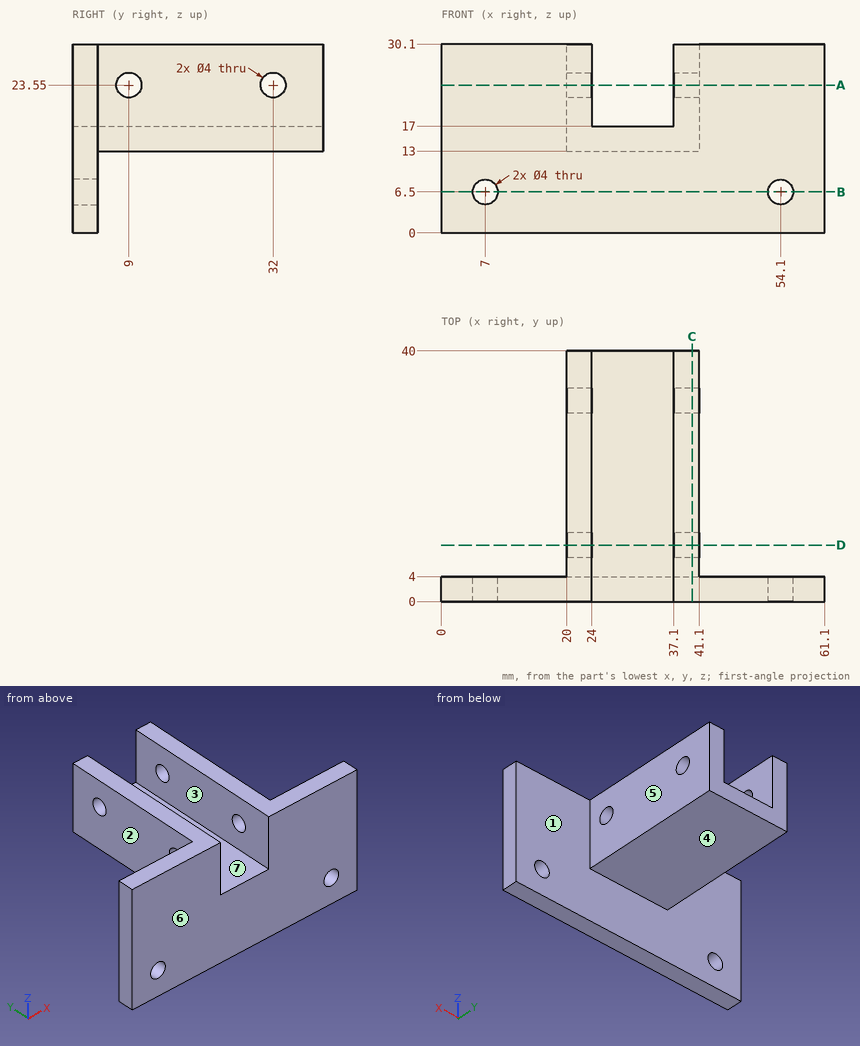
Geometry: see drawing. Coordinates: mm, zero at the bounding-box minimum. A direction names the side the tool comes from. Give positions to 0.01 mm unless a question says otherwise; leave off trailing zeros. Loops run counter-clockwise (first coordinate to the right, second up) from the corner with the lowest first, then second, coordinate; pieces in that order, holes last. Notation, with made-up numbers: (36, 84) - (79, 84) arc R12 cw to (79, 102) - close; hole circle Ø5 at (20.25, 26). An arc over 180 degrees is marked (long way). Use CSV: the item, a comma, the result in double quotes.
1) Mould query, pull axis X, two halves, no side actions, for the marked faces 5, 6 and 7. Classes: +X half, -X half, draft (parallel to the pull), parting line (faces both ways), or undercut.
Worked out:
face 5,"+X half"
face 6,"draft"
face 7,"undercut"
2) Cut plane D-D (y = 9). Output: boundary loops of the cut face in (x, z).
Worked out:
outline,"(20, 13) - (41.1, 13) - (41.1, 21.55) - (37.1, 21.55) - (37.1, 17) - (24, 17) - (24, 21.55) - (20, 21.55) - close; (20, 25.55) - (24, 25.55) - (24, 30.1) - (20, 30.1) - close; (37.1, 25.55) - (41.1, 25.55) - (41.1, 30.1) - (37.1, 30.1) - close"
3) Set-up query: the marked faces 1, 2, 3 and 4. Return all of +Z, -Z, +X, -X, +Y, -Y with unobstructed straight access to the full face (end or side cutting, diameter ignored); none if empty.
Worked out:
face 1,"-Z, +Y"
face 2,"+Z, -Z, -X, +Y"
face 3,"+Z, +Y, -Y"
face 4,"-Z, +X, -X, +Y"
4) Line query: line 1 (Y direction, x = 22.95, z = 23.55); line 2 (X direction, y = 3.05, z = 6.5); line 3 (Y direction, x = 39, z = 23). Output: solid intervals per line, ascending.
Worked out:
line 1,"y = 0 to 7, 11 to 30, 34 to 40"
line 2,"x = 0 to 5, 9 to 52.1, 56.1 to 61.1"
line 3,"y = 0 to 7.08, 10.92 to 30.08, 33.92 to 40"
5) Cut plane A-A (z = 23.55). Output: boundary loops of the cut face in (x, y), and give its area (3 significant figures).
Worked out:
outline,"(0, 0) - (24, 0) - (24, 7) - (20, 7) - (20, 4) - (0, 4) - close; (20, 11) - (24, 11) - (24, 30) - (20, 30) - close; (20, 34) - (24, 34) - (24, 40) - (20, 40) - close; (37.1, 0) - (61.1, 0) - (61.1, 4) - (41.1, 4) - (41.1, 7) - (37.1, 7) - close; (37.1, 11) - (41.1, 11) - (41.1, 30) - (37.1, 30) - close; (37.1, 34) - (41.1, 34) - (41.1, 40) - (37.1, 40) - close"
area,"416 mm^2"
6) Pin query (flat end, axial travel): P1, Ø5, axis at y = 14, z = 25.5, coming from the +X side; P2, Ø10.5, axis at x = 26.5, y = 16, coming from the -Z side; P3, Ø3.5, axis at y = 9, z = 23.55, coming from the -X side; P4, Ø6.5, axis at y = 32, z = 23.55, coming from the -X side. Return the tip coordinate at first contact, or that it passes through.
Worked out:
P1,"stops at x = 41.1"
P2,"stops at z = 13"
P3,"passes through"
P4,"stops at x = 20"
7) Cut plane C-C (x = 40). Output: boundary loops of the cut face in (y, z).
Worked out:
outline,"(0, 0) - (4, 0) - (4, 13) - (40, 13) - (40, 30.1) - (0, 30.1) - close; hole circle Ø4 at (9, 23.55); hole circle Ø4 at (32, 23.55)"
8) Cut plane B-B (z = 6.5). Output: boundary loops of the cut face in (x, y).
Worked out:
outline,"(0, 0) - (5, 0) - (5, 4) - (0, 4) - close; (9, 0) - (52.1, 0) - (52.1, 4) - (9, 4) - close; (56.1, 0) - (61.1, 0) - (61.1, 4) - (56.1, 4) - close"
